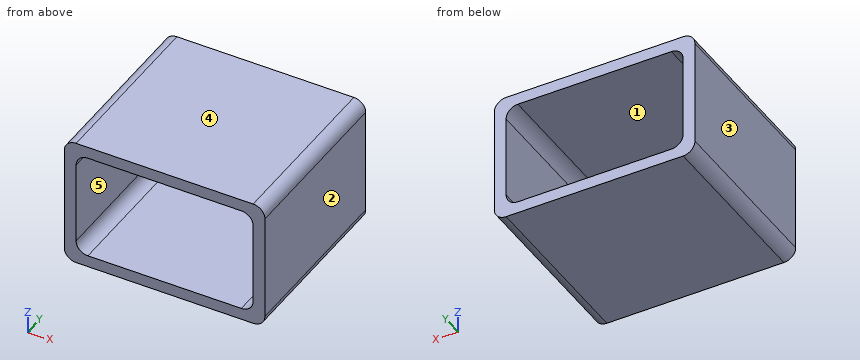
```python
from build123d import *

# Parameters (mm, degrees)
F1_DEPTH      = 9.525
F1_DEPTH_BACK = 9.525


with BuildPart() as f1:
    # F0 (on Front) → F1 (new body, two sides)
    with BuildSketch(Plane.XZ) as f1_sk:
        with BuildLine():
            Line((-9.525, -6.985), (9.525, -6.985))
            ThreePointArc((9.525, -6.985), (10.423026, -6.613026), (10.795, -5.715))
            Line((10.795, -5.715), (10.795, 5.715))
            ThreePointArc((10.795, 5.715), (10.423026, 6.613026), (9.525, 6.985))
            Line((9.525, 6.985), (-9.525, 6.985))
            ThreePointArc((-9.525, 6.985), (-10.423026, 6.613026), (-10.795, 5.715))
            Line((-10.795, 5.715), (-10.795, -5.715))
            ThreePointArc((-10.795, -5.715), (-10.423026, -6.613026), (-9.525, -6.985))
        make_face()
        with BuildLine():
            ThreePointArc((9.525, -4.445), (9.153026, -5.343026), (8.255, -5.715))
            Line((8.255, -5.715), (-8.255, -5.715))
            ThreePointArc((-8.255, -5.715), (-9.153026, -5.343026), (-9.525, -4.445))
            Line((-9.525, -4.445), (-9.525, 4.445))
            ThreePointArc((-9.525, 4.445), (-9.153026, 5.343026), (-8.255, 5.715))
            Line((-8.255, 5.715), (8.255, 5.715))
            ThreePointArc((8.255, 5.715), (9.153026, 5.343026), (9.525, 4.445))
            Line((9.525, 4.445), (9.525, -4.445))
        make_face(mode=Mode.SUBTRACT)
    extrude(amount=F1_DEPTH)
    extrude(f1_sk.sketch, amount=-F1_DEPTH_BACK)


solid = f1.part
```
The model under review builds one solid part; all positions refer to its coordinate system, in mm. Face numbers are marked on the shaded views. A direction names the side the tool comes from. Round coordinates to 2 decimals unless told otherwise and drop trailing zeros. Loops run counter-clockwise (first coordinate to the right, second up) from the corner with the lowest first, then second, coordinate; pieces in that order, holes last. Notation, with made-up numbers: M 84.5,-39 L 116.5,-39 A17 ccw 116.5,-34 Z; hole C -9.5,63.5 d6. An arc over 180 degrees is marked long. Write item = value, one per line.
Item 1: Take a section at A-A on x = -6.25. Write out the cut boundary in (y, z) (3 decimals), then the cut area to 3 significant figures.
Return value:
outline = M -9.525,-6.985 L 9.525,-6.985 L 9.525,-5.715 L -9.525,-5.715 Z; M -9.525,5.715 L 9.525,5.715 L 9.525,6.985 L -9.525,6.985 Z
area = 48.4 mm2
Item 2: The part is to be moulded in two halves that separate along X. For the marked faces 3, 4 and 5, say which applies: released by +X, released by -X, zero draft, split by the parting line, or undercut.
Return value:
face_3 = released by -X
face_4 = zero draft
face_5 = undercut
Item 3: Machinability: for the marked faces 1 and 2, which of the approach directions +Z, -Z, +X, -X, +Y, -Y give a long, thin tool a straight path to every point of the face, cutting with its end or side? Answer none if there is none.
Return value:
face_1 = +Y, -Y
face_2 = +Z, -Z, +X, +Y, -Y
Item 4: Take a section at B-B on y = -4.25. Write out the cut boundary in (x, z) (3 decimals).
Return value:
outline = M -10.795,-5.715 A1.27 ccw -9.525,-6.985 L 9.525,-6.985 A1.27 ccw 10.795,-5.715 L 10.795,5.715 A1.27 ccw 9.525,6.985 L -9.525,6.985 A1.27 ccw -10.795,5.715 Z; hole M -9.525,-4.445 A1.27 ccw -8.255,-5.715 L 8.255,-5.715 A1.27 ccw 9.525,-4.445 L 9.525,4.445 A1.27 ccw 8.255,5.715 L -8.255,5.715 A1.27 ccw -9.525,4.445 Z
Item 5: For line 1 (X direction, y = 6.75, z = -1.5) (3 decimals); line 2 (Z direction, x = -7, y = -0.5) (3 decimals); line 3 (X direction, y = -7.25, z = -5.5) (3 decimals), list the stretches that pass through material, from the lowest coordinate up. Write a range as [from, to].
Return value:
line_1 = [-10.795, -9.525], [9.525, 10.795]
line_2 = [-6.985, -5.715], [5.715, 6.985]
line_3 = [-10.795, -8.962], [8.962, 10.795]
Item 6: Take a section at C-C on z = -3.25. Write out the cut boundary in (x, y) (3 decimals).
Return value:
outline = M -10.795,-9.525 L -9.525,-9.525 L -9.525,9.525 L -10.795,9.525 Z; M 9.525,-9.525 L 10.795,-9.525 L 10.795,9.525 L 9.525,9.525 Z
